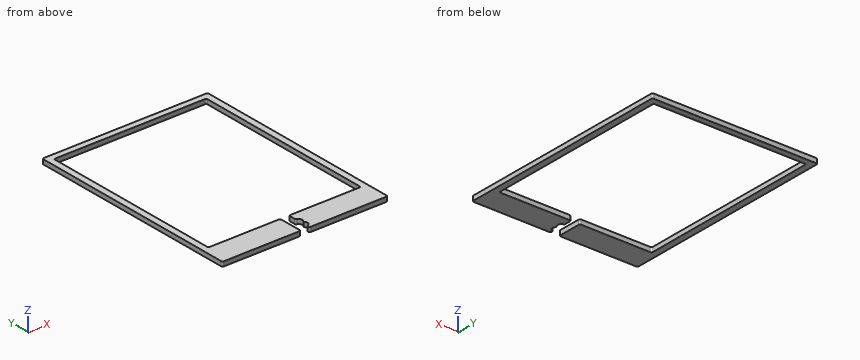
```python
from build123d import *

# Parameters (mm, degrees)
F1_DEPTH = 6.35
F2_R     = 2


# Not quite as in the source:
# - a length typed as a fraction of an inch, garbled in the dataset ("3 / 203.2 mm" for 3/8 in), is restored


with BuildPart() as f1:
    # F0 (on Top) → F1 (new body)
    with BuildSketch(Plane.XY):
        with BuildLine():
            Line((115, -150.5), (115, 150.5))
            Line((115, 150.5), (-115, 150.5))
            Line((-115, 150.5), (-115, -150.5))
            Line((-115, -150.5), (-6, -150.5))
            Line((-6, -150.5), (-6, -116.2))
            Line((-6, -116.2), (-106, -116.2))
            Line((-106, -116.2), (-106, 141.8))
            Line((-106, 141.8), (106, 141.8))
            Line((106, 141.8), (106, -116.2))
            Line((106, -116.2), (6, -116.2))
            Line((6, -116.2), (6, -127.5))
            ThreePointArc((6, -127.5), (10.8733971724, -131.3819660113), (8.1794494718, -137))
            ThreePointArc((8.1794494718, -137), (10.8733971724, -142.6180339887), (6, -146.5))
            Line((6, -146.5), (6, -150.5))
            Line((6, -150.5), (115, -150.5))
        make_face()
    extrude(amount=F1_DEPTH)

    # F2
    f2_edges = [f1.edges().sort_by_distance(p)[0] for p in [
        (115, -150.5, 3.175),
        (115, 150.5, 3.175),
        (6, -116.2, 3.175),
        (-6, -116.2, 3.175),
        (-6, -150.5, 3.175),
        (-106, -116.2, 3.175),
        (-115, 150.5, 3.175),
        (6, -127.5, 3.175),
        (8.179449, -137, 3.175),
        (6, -146.5, 3.175),
        (-115, -150.5, 3.175),
        (106, 141.8, 3.175),
        (106, -116.2, 3.175),
        (-106, 141.8, 3.175),
        (6, -150.5, 3.175),
    ]]
    fillet(f2_edges, radius=F2_R)


solid = f1.part
```
The listing builds one solid part. Answer for the finished solid, in the listing's coordinates (mm). Coordinates: 2 decimals unless noted, no trailing zeros. Write each loop counter-clockwise with the first axis right and the second up, starting at its lowest first coordinate (ties: lowest second). Pieces come first, ordered by that corner, then holes. Notation, with made-up numbers: (80, -35.75) - (131, -35.75) arc R30 ccw to (131, -12.75) - close; hole circle Ø4 at (76, 22). An arc over 180 degrees is marked (long way). Return JSON: item names as keys, results as strings. Group by question number.
1. A cutting plane is placed at B-B, the plane y = -90.5. Determine the outline of the cut face in (x, z), plus the area to 3 significant figures.
2. Straight lines are drawn through the part: L1, parallel to X at y = -118.5, z = 1.5; L2, parallel to X at y = -33, z = 6; L3, parallel to Y at x = -24, z = 2. For each, find the intervals that lie inside material, in ascending order.
3. A cutting plane is placed at A-A, the plane x = -15. Determine the outline of the cut face in (y, z).
Ans:
{
 "1": {"outline": "(-115, 0) - (-106, 0) - (-106, 6.35) - (-115, 6.35) - close; (106, 0) - (115, 0) - (115, 6.35) - (106, 6.35) - close", "area": "114 mm²"},
 "2": {"L1": "-115 to -6, 6 to 115", "L2": "-115 to -106, 106 to 115", "L3": "-150.5 to -116.2, 141.8 to 150.5"},
 "3": {"outline": "(-150.5, 0) - (-116.2, 0) - (-116.2, 6.35) - (-150.5, 6.35) - close; (141.8, 0) - (150.5, 0) - (150.5, 6.35) - (141.8, 6.35) - close"}
}
